```python
from build123d import *

# Parameters (mm, degrees)
BOSS_EXTRUDE1_DEPTH      = 13
BOSS_EXTRUDE1_DEPTH_BACK = 13
SKETCH1_W                = 53
SKETCH1_H                = 5
SKETCH2_W                = 7
SKETCH2_H                = 11.1
BOSS_EXTRUDE2_DEPTH      = 26
CUT_EXTRUDE1_DEPTH       = 8
CUT_EXTRUDE1_DEPTH_BACK  = 8
SKETCH3_W                = 7
SKETCH3_H                = 11.1
CUT_EXTRUDE3_START       = -26.000001
CUT_EXTRUDE3_DEPTH       = 26.000002
CUT_EXTRUDE5_REACH       = 62.068
SKETCH6_R                = 1.25
SKETCH7_W                = 50
SKETCH7_H                = 7.11
BOSS_EXTRUDE3_DEPTH      = 0.5


with BuildPart() as part:
    # Sketch1 → Boss-Extrude1 (new, two sides: drawn at the far end of the back side and taken through both)
    with BuildSketch(Plane.XY.offset(-BOSS_EXTRUDE1_DEPTH_BACK)):
        with Locations((26.5, 2.5)):
            Rectangle(SKETCH1_W, SKETCH1_H)
    extrude(amount=BOSS_EXTRUDE1_DEPTH + BOSS_EXTRUDE1_DEPTH_BACK)

    # Sketch2 → Boss-Extrude2 (add)
    with BuildSketch(Plane.XY.offset(13)):
        with Locations((-3.5, 5.55)):
            Rectangle(SKETCH2_W, SKETCH2_H)
    extrude(amount=-BOSS_EXTRUDE2_DEPTH)

    # Sketch3 → Cut-Extrude1 (cut, two sides: drawn at the far end of the back side and taken through both)
    with BuildSketch(Plane.XY.offset(-CUT_EXTRUDE1_DEPTH_BACK)):
        with Locations((-3.5, 5.55)):
            Rectangle(SKETCH3_W, SKETCH3_H)
    extrude(amount=CUT_EXTRUDE1_DEPTH + CUT_EXTRUDE1_DEPTH_BACK, mode=Mode.SUBTRACT)

    # Sketch5 → Cut-Extrude3 (cut)
    with BuildSketch(Plane.XY.offset(13).offset(CUT_EXTRUDE3_START)):
        with BuildLine():
            Line((-7, 0), (-2.615264285, 0))
            ThreePointArc((-2.615264285, 0), (-5.774039172, 2.011497403), (-7, 5.55))
            Line((-7, 5.55), (-7, 0))
        make_face()
    extrude(amount=CUT_EXTRUDE3_DEPTH, mode=Mode.SUBTRACT)

    # Cut-Extrude5: up to this face of the body (flat: up to its plane)
    cut_extrude5_end = Plane(part.part.faces().sort_by_distance((20.170778463, 3.227224149, -13))[0])
    # Sketch6 → Cut-Extrude5 (cut, up to the picked face)
    with BuildSketch(Plane.XY.offset(13), mode=Mode.PRIVATE) as cut_extrude5_sk1:
        with Locations(Location((-3.5, 5.55, 0), (0, 0, 180))):
            Circle(SKETCH6_R)
    cut_extrude5_tool1 = split(extrude(cut_extrude5_sk1.sketch, amount=-CUT_EXTRUDE5_REACH, mode=Mode.PRIVATE), bisect_by=cut_extrude5_end, keep=Keep.BOTH, mode=Mode.PRIVATE)
    add(cut_extrude5_tool1.solids().sort_by(Axis((-3.5, 5.55, 13), (0, 0, -1)))[0], mode=Mode.SUBTRACT)

    # Sketch7 → Boss-Extrude3 (add)
    with BuildSketch(Plane.XZ):
        with Locations((26.5, 0)):
            Rectangle(SKETCH7_W, SKETCH7_H)
    extrude(amount=BOSS_EXTRUDE3_DEPTH)


solid = part.part
```
CAD build for the part. Positions are in the model's coordinates, mm. A direction names the side the tool comes from. Coordinates: 2 decimals unless noted, no trailing zeros. Order: outer loops, then holes, each group sorted by start corner. A loop starts at its lowest first (then second) coordinate and runs counter-clockwise, first axis right, second up. Notation, with made-up numbers: (62.25, -0.75) -> (116.25, -0.75) arc R25 cw to (116.25, 29.25) -> close; hole circle Ø4 at (-16, 49.5). An arc over 180 degrees is marked (long way). Use one line per item in the form item = value. Start each with the question number.
1) Band-saw the part on C-C on x = 3.5. Give the cut face in (y, z) (3 decimals), then the cut area to 3 significant figures.
2) Drop flat-ended pins along their axis: pin 1 (4 mm diameter, centred on x = 26, z = 8, fed in from -Y); pin 2 (1.5 mm diameter, centred on y = 8, z = -10, fed in from +X); pin 3 (0.6 mm diameter, centred on x = 35, y = -0.5, fed in from +Z) (3 decimals). Give the stop position or say it passes through.
3) Drill centre lines: L1, parallel to X at y = 5.55, z = 10.4; L2, parallel to Z at x = -1.5, y = 6.5; L3, parallel to X at y = 4, z = 3. Where is each one in solid material? Low to high. Write a range as [from, to].
4) Pull direction X, two halves, no side cores. Call faces 4 (the cylindrical face through (-4.7, 5.2, 10.5)), 5 (the flat face through (-7, 8, 11)), 6 (the flat face through (25, 0, 6)): +X half, -X half, draft (parallel to the pull), parting line (faces both ways), or undercut.
5) Band-saw the part on A-A on y = 8.25. Give the cut face in (x, z), then the cut area to 3 significant figures.
6) Band-saw the part on D-D on z = -3. Give the cut face in (x, y).
7) Tool access for faces 1 (the flat face through (26, 5, 0)), 2 (the cylindrical face through (-5.735, 1.963, 10.465)), 3 (the flat face through (-4, 7, -8)): list every direction of +Z, -Z, +X, -X, +Y, -Y with a clear straight run to the whole face (end or side of a thin tool).
8) Band-saw the part on B-B on z = 8.75. Give the cut face in (x, y), then the cut area to 3 significant figures.
Entries:
q1.outline = (-0.5, -3.555) -> (0, -3.555) -> (0, -13) -> (5, -13) -> (5, 13) -> (0, 13) -> (0, 3.555) -> (-0.5, 3.555) -> close
q1.area = 134 mm2
q2.pin_1 = 0
q2.pin_2 = 0
q2.pin_3 = 3.555
q3.L1 = [-7, -4.75], [-2.25, 0]
q3.L2 = [-13, -8], [8, 13]
q3.L3 = [0, 53]
q4.face_4 = undercut
q4.face_5 = -X half
q4.face_6 = draft
q5.outline = (-7, -13) -> (0, -13) -> (0, -8) -> (-7, -8) -> close; (-7, 8) -> (0, 8) -> (0, 13) -> (-7, 13) -> close
q5.area = 70.0 mm2
q6.outline = (0, 0) -> (1.5, 0) -> (1.5, -0.5) -> (51.5, -0.5) -> (51.5, 0) -> (53, 0) -> (53, 5) -> (0, 5) -> close
q7.face_1 = +Z, -Z, +X, +Y
q7.face_2 = +Z, -Z, -X, -Y
q7.face_3 = -X, +Y, -Y
q8.outline = (-7, 5.53) arc R5.69 ccw to (-2.62, 0) -> (53, 0) -> (53, 5) -> (0, 5) -> (0, 11.1) -> (-7, 11.1) -> close; hole circle Ø2.5 at (-3.5, 5.55)
q8.area = 332 mm2
